from build123d import *

# Parameters (mm, degrees)
BOSS_EXTRUDE1_START      = -4
BOSS_EXTRUDE1_DEPTH      = 8
M3_CLEARANCE_HOLE1_D     = 3.2
M3_CLEARANCE_HOLE1_DEPTH = 8.8


with BuildPart() as part:
    # Sketch2 → Boss-Extrude1 (new body)
    with BuildSketch(Plane(origin=(0, 0, 0), x_dir=(1, 0, 0), z_dir=(0, 1, 0)).offset(BOSS_EXTRUDE1_START)):
        with BuildLine():
            ThreePointArc((-7.729285786, -6.5), (-6.095063245, -7.609772229), (-4.158571571, -8))
            Line((-4.158571571, -8), (4.158571571, -8))
            ThreePointArc((4.158571571, -8), (6.095063245, -7.609772229), (7.729285786, -6.5))
            ThreePointArc((7.729285786, -6.5), (9.363508327, -5.390227771), (11.3, -5))
            Line((11.3, -5), (12.3, -5))
            Line((12.3, -5), (12.3, 0))
            Line((12.3, 0), (11.3, 0))
            Line((11.3, 0), (3.5, 0))
            Line((3.5, 0), (3.5, -3.407197308))
            Line((3.5, -3.407197308), (-3.5, -3.407197308))
            Line((-3.5, -3.407197308), (-3.5, 0))
            Line((-3.5, 0), (-11.3, 0))
            Line((-11.3, 0), (-12.3, 0))
            Line((-12.3, 0), (-12.3, -5))
            Line((-12.3, -5), (-11.3, -5))
            ThreePointArc((-11.3, -5), (-9.363508327, -5.390227771), (-7.729285786, -6.5))
        make_face()
    extrude(amount=BOSS_EXTRUDE1_DEPTH)

    # M3 Clearance Hole1
    with Locations(Plane.ZY.offset(12.3)):
        with Locations((2.5, 0)):
            m3_clearance_hole1 = Hole(M3_CLEARANCE_HOLE1_D / 2, depth=M3_CLEARANCE_HOLE1_DEPTH)

    # Mirror1: M3 Clearance Hole1 across plane
    add(m3_clearance_hole1.mirror(Plane(origin=(0, 0, 0), x_dir=(0, 0, 1), z_dir=(1, 0, 0))), mode=Mode.SUBTRACT)


solid = part.part
The listing builds one solid part. Answer for the finished solid, in the listing's coordinates (mm). A direction names the side the tool comes from. Give positions to 0.01 mm unless a question says otherwise; leave off trailing zeros. Loops run counter-clockwise (first coordinate to the right, second up) from the corner with the lowest first, then second, coordinate; pieces in that order, holes last. Notation, with made-up numbers: (-37.75, 5) - (3.25, 5) arc R23 cw to (3.25, 20) - close; hole circle Ø3 at (59, -3.75). An arc over 180 degrees is marked (long way). Answer as a JSON object with one key per item and string values.
1. A cutting plane is placed at D-D (x = 1.5). Write down the section's boundary in (y, z).
Determined:
{"outline": "(-4, 3.41) - (4, 3.41) - (4, 8) - (-4, 8) - close"}
2. Find the intervals of material crossed by L1, parallel to Y at x = 7.25, z = 2.5; L2, parallel to X at y = -0.75, z = 1; L3, parallel to Z at x = 5.75, y = 0, in increasing order. Write a range as [from, to].
Determined:
{"L1": "[-4, -1.6], [1.6, 4]", "L2": "[-12.3, -3.5], [3.5, 12.3]", "L3": "[0, 0.9], [4.1, 7.74]"}
3. A cutting plane is placed at C-C (y = 3.25). Write down the section's boundary in (x, z).
Determined:
{"outline": "(-12.3, 0) - (-3.5, 0) - (-3.5, 3.41) - (3.5, 3.41) - (3.5, 0) - (12.3, 0) - (12.3, 5) - (11.3, 5) arc R5 cw to (7.73, 6.5) arc R5 ccw to (4.16, 8) - (-4.16, 8) arc R5 ccw to (-7.73, 6.5) arc R5 cw to (-11.3, 5) - (-12.3, 5) - close"}
4. Flat-ended cylindrical pins translate along their axes: pin 1 Ø3.5 at (x, y) = (-1.5, -1.5) entering from -Z; pin 2 Ø2 at (x, z) = (1, 1) entering from +Y; pin 3 Ø2.5 at (y, z) = (0, 2.5) entering from +X; pin 4 Ø0.8 at (x, y) = (-12, 2) entering from +Z. Find the tip coordinate at first contact, or state that the pin passes through.
Determined:
{"pin 1": "z = 3.41", "pin 2": "through", "pin 3": "x = 3.5", "pin 4": "z = 5"}
5. For a pull along Z with two mould halves and no side action, classify faces 1 (the flat face through (-12.3, 2, 2)), 2 (the flat face through (0, 0, 8)), 3 (the cylindrical face through (7.838, 0.481, 0.974)) as pulls with the +Z half, pulls with the -Z half, needs draft (parallel to the pull), parting line crosses it, or undercut.
Determined:
{"face 1": "needs draft", "face 2": "pulls with the +Z half", "face 3": "undercut"}
6. For faces 4 (the flat face through (-12, 0, 5)), 5 (the flat face through (12, 0, 5)), 6 (the flat face through (-8, 0, 0)), 7 (the flat face through (3.5, -0.1, 0.5)), 8 (the cylindrical face through (-7.838, 0.481, 0.974)), determine the directions among +Z, -Z, +X, -X, +Y, -Y from which every point of the face is accessible in a straight line to the end or side of a thin tool.
Determined:
{"face 4": "+Z, -X, +Y, -Y", "face 5": "+Z, +X, +Y, -Y", "face 6": "-Z, +X, -X, +Y, -Y", "face 7": "-Z, +Y, -Y", "face 8": "-X"}
7. A cutting plane is placed at A-A (y = 0). Write down the section's boundary in (x, z), then the cut area to 3 significant figures.
Determined:
{"outline": "(-12.3, 0) - (-3.5, 0) - (-3.5, 0.9) - (-12.3, 0.9) - close; (-12.3, 4.1) - (-3.5, 4.1) - (-3.5, 3.41) - (3.5, 3.41) - (3.5, 4.1) - (12.3, 4.1) - (12.3, 5) - (11.3, 5) arc R5 cw to (7.73, 6.5) arc R5 ccw to (4.16, 8) - (-4.16, 8) arc R5 ccw to (-7.73, 6.5) arc R5 cw to (-11.3, 5) - (-12.3, 5) - close; (3.5, 0) - (12.3, 0) - (12.3, 0.9) - (3.5, 0.9) - close", "area": "89.2 mm²"}
8. A cutting plane is placed at B-B (z = 2.5). Write down the section's boundary in (x, y), then the cut area to 3 significant figures.
Determined:
{"outline": "(-12.3, -4) - (-3.5, -4) - (-3.5, -1.6) - (-12.3, -1.6) - close; (-12.3, 1.6) - (-3.5, 1.6) - (-3.5, 4) - (-12.3, 4) - close; (3.5, -4) - (12.3, -4) - (12.3, -1.6) - (3.5, -1.6) - close; (3.5, 1.6) - (12.3, 1.6) - (12.3, 4) - (3.5, 4) - close", "area": "84.5 mm²"}
